```python
from build123d import *

# Parameters (mm, degrees)
SKETCH1_R               = 2.5
BOSS_EXTRUDE1_DEPTH     = 20
CUT_EXTRUDE1_DEPTH      = 56.523080786
CUT_EXTRUDE1_DEPTH_BACK = 56.523080786
SKETCH2_W               = 16
SKETCH2_H               = 47.239813723
SKETCH2_H_2             = 47.470835296


with BuildPart() as part:
    # Sketch1 → Boss-Extrude1 (new body)
    with BuildSketch(Plane(origin=(0, 0, 0), x_dir=(0, 0, -1), z_dir=(1, 0, 0))):
        with BuildLine():
            Line((47.5, 3.75), (-47.5, 3.75))
            ThreePointArc((-47.5, 3.75), (-51.25, 0), (-47.5, -3.75))
            Line((-47.5, -3.75), (47.5, -3.75))
            ThreePointArc((47.5, -3.75), (51.25, 0), (47.5, 3.75))
        make_face()
        with Locations((-47.5, 0)):
            Circle(SKETCH1_R, mode=Mode.SUBTRACT)
        with Locations((47.5, 0)):
            Circle(SKETCH1_R, mode=Mode.SUBTRACT)
    extrude(amount=BOSS_EXTRUDE1_DEPTH)

    # Sketch2 → Cut-Extrude1 (cut, two sides: drawn at the far end of the back side and taken through both)
    with BuildSketch(Plane(origin=(0, 3.75, 0), x_dir=(1, 0, 0), z_dir=(0, 1, 0)).offset(-CUT_EXTRUDE1_DEPTH_BACK)):
        with Locations((10, 27.630093139)):
            Rectangle(SKETCH2_W, SKETCH2_H)
        with Locations((10, -27.514582352)):
            Rectangle(SKETCH2_W, SKETCH2_H_2)
    extrude(amount=CUT_EXTRUDE1_DEPTH + CUT_EXTRUDE1_DEPTH_BACK, mode=Mode.SUBTRACT)


solid = part.part
```
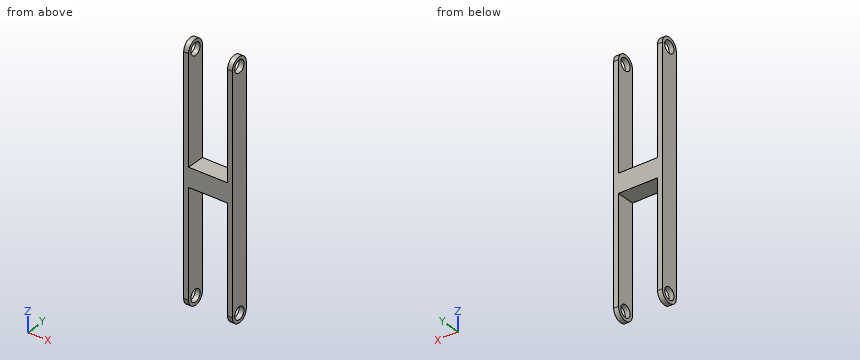
For this review, take the finished solid that the model builds, in its own axes (mm). Coordinates: 2 decimals unless noted, no trailing zeros. Order: outer loops, then holes, each group sorted by start corner. A loop starts at its lowest first (then second) coordinate and runs counter-clockwise, first axis right, second up. Notation, with made-up numbers: (24.25, 68) - (72.25, 68) arc R11 cw to (72.25, 77) - close; hole circle Ø4 at (-1, 69). An arc over 180 degrees is marked (long way). Answer as a JSON object with one key per item and string values. Group by question number.
1. We need section B-B on z = -9.5. State the section outline as (x, y) points, then the cut area to 3 significant figures.
2. For probe 1 along Z at (x, y) = (1.55, 0); probe 2 along Y at (x, z) = (1.05, 47.5); probe 3 along X at (y, z) = (0.75, 7), list the stretches that pass through material, from the lowest coordinate up.
3. Clearance check with flat-ended pins moving along their axes: P1, Ø4, axis at y = 1.5, z = -33, coming from the -X side; P2, Ø3, axis at y = 0, z = -47.5, coming from the +X side; P3, Ø1, axis at x = 8.5, y = 1.5, coming from the -Z side; P4, Ø1, axis at x = 14, y = 2, coming from the +Z side. State where each tip first meets the part, or that it passes through.
4. We need section C-C on x = 17. State the section outline as (y, z) points, then the cut area to 3 significant figures.
5. We need section A-A on y = 0. State the section outline as (x, z) points, then the cut area to 3 significant figures.
Final values:
{
 "1": {"outline": "(0, -3.75) - (2, -3.75) - (2, 3.75) - (0, 3.75) - close; (18, -3.75) - (20, -3.75) - (20, 3.75) - (18, 3.75) - close", "area": "30.0 mm²"},
 "2": {"probe 1": "-51.25 to -50, -45 to 45, 50 to 51.25", "probe 2": "-3.75 to -2.5, 2.5 to 3.75", "probe 3": "0 to 2, 18 to 20"},
 "3": {"P1": "x = 0", "P2": "through", "P3": "z = -4.01", "P4": "z = 3.78"},
 "4": {"outline": "(-3.75, -4.01) - (3.75, -4.01) - (3.75, 3.78) - (-3.75, 3.78) - close", "area": "58.4 mm²"},
 "5": {"outline": "(0, -51.25) - (2, -51.25) - (2, -50) - (0, -50) - close; (0, -45) - (2, -45) - (2, -4.01) - (18, -4.01) - (18, -45) - (20, -45) - (20, 45) - (18, 45) - (18, 3.78) - (2, 3.78) - (2, 45) - (0, 45) - close; (0, 50) - (2, 50) - (2, 51.25) - (0, 51.25) - close; (18, -51.25) - (20, -51.25) - (20, -50) - (18, -50) - close; (18, 50) - (20, 50) - (20, 51.25) - (18, 51.25) - close", "area": "495 mm²"}
}
